The drawing under review shows one solid part. Ordinate dimensions are in mm from its lowest x, y, z. A direction names the side the tool comes from. Coordinates: 2 decimals unless noted, no trailing zeros. Order: outer loops, then holes, each group sorted by start corner. A loop starts at its lowest first (then second) coordinate and runs counter-clockwise, first axis right, second up. Notation, with made-up numbers: (14.25, 64) -> (47.25, 64) arc R32 ccw to (47.25, 96) -> close; hole circle Ø3 at (-0.75, 86.5). An arc over 180 degrees is marked (long way). Put each result on its own line as item: value.
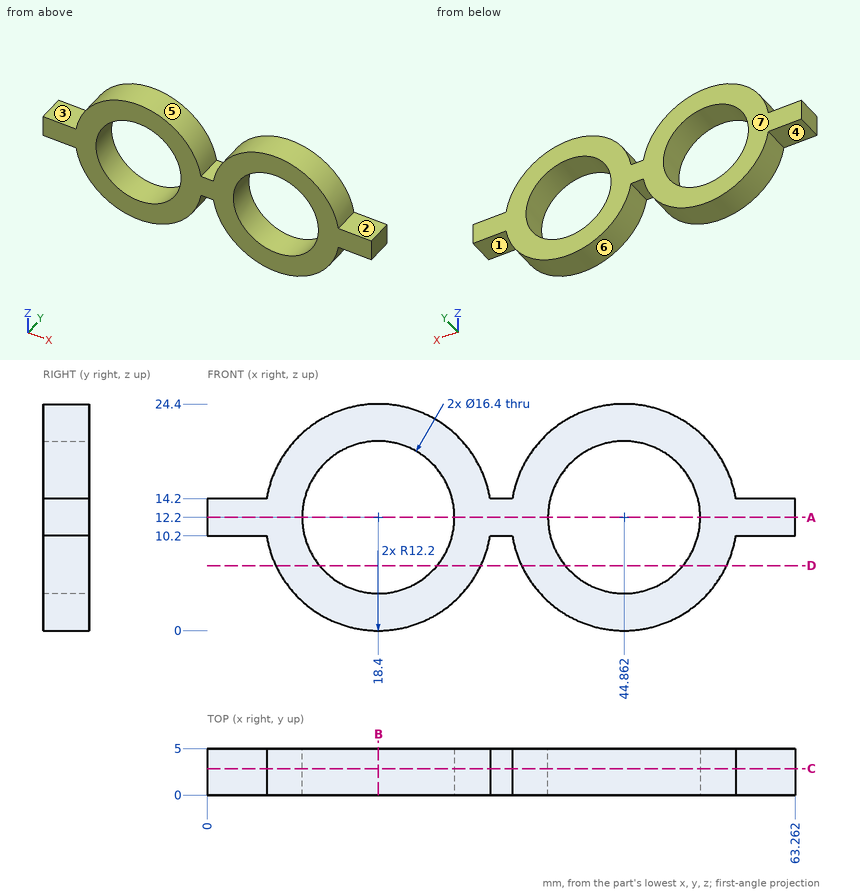
Item 1: For line 1 (X direction, y = 2.75, z = 6.5); line 2 (X direction, y = 0.2, z = 15.25); line 3 (X direction, y = 1.7, z = 13.5), list the stretches that pass through material, from the lowest coordinate up. Write a range as from..to.
Answers below:
line 1: 7.61..12.51, 24.29..29.19, 34.08..38.97, 50.76..55.65
line 2: 6.59..10.79, 26.01..30.21, 33.05..37.25, 52.47..56.67
line 3: 0..10.3, 26.5..36.77, 52.96..63.26
Item 2: Consider section A-A on z = 12.2. Write out the cut boundary in (x, y), and give its area (3 significant figures).
Answers below:
outline: (0, 0) -> (10.2, 0) -> (10.2, 5) -> (0, 5) -> close; (26.6, 0) -> (36.66, 0) -> (36.66, 5) -> (26.6, 5) -> close; (53.06, 0) -> (63.26, 0) -> (63.26, 5) -> (53.06, 5) -> close
area: 152 mm^2
Item 3: Consider section C-C on y = 2.85. Write out the cut boundary in (x, z).
Answers below:
outline: (0, 10.2) -> (6.37, 10.2) arc R12.2 ccw to (30.43, 10.2) -> (32.83, 10.2) arc R12.2 ccw to (56.9, 10.2) -> (63.26, 10.2) -> (63.26, 14.2) -> (56.9, 14.2) arc R12.2 ccw to (32.83, 14.2) -> (30.43, 14.2) arc R12.2 ccw to (6.37, 14.2) -> (0, 14.2) -> close; hole circle Ø16.4 at (18.4, 12.2); hole circle Ø16.4 at (44.86, 12.2)
Item 4: Consider section D-D on z = 7. Write out the cut boundary in (x, y), and give its area (3 significant figures).
Answers below:
outline: (7.36, 0) -> (12.06, 0) -> (12.06, 5) -> (7.36, 5) -> close; (24.74, 0) -> (29.44, 0) -> (29.44, 5) -> (24.74, 5) -> close; (33.83, 0) -> (38.52, 0) -> (38.52, 5) -> (33.83, 5) -> close; (51.2, 0) -> (55.9, 0) -> (55.9, 5) -> (51.2, 5) -> close
area: 93.9 mm^2
Item 5: Mouldability with a two-part tool opening along X and no side actions: class the marked faces 5, 6 and 7 as +X half, -X half, draft (parallel to the pull), parting line (faces both ways), or undercut.
Answers below:
face 5: undercut
face 6: undercut
face 7: draft
Item 6: For the marked faces 1, 2, 3 and 4, list the 3-axis set-ups (+Z, -Z, +X, -X, +Y, -Y) from which the entire face can be reached by the end or side of a thin tool; tool diameter is ignored.
Answers below:
face 1: -Z, +X, +Y, -Y
face 2: +Z, +X, +Y, -Y
face 3: +Z, -X, +Y, -Y
face 4: -Z, -X, +Y, -Y
Item 7: Consider section B-B on x = 18.4. Write out the cut boundary in (y, z), and give its area (3 significant figures).
Answers below:
outline: (0, 0) -> (5, 0) -> (5, 4) -> (0, 4) -> close; (0, 20.4) -> (5, 20.4) -> (5, 24.4) -> (0, 24.4) -> close
area: 40.0 mm^2
Item 8: For pin 1 Ø2 at (x, y) = (52.5, 1) entering from +Z; pin 2 Ø1.5 at (y, z) = (2.5, 5.5) entering from -X; pin 3 Ø1.9 at (x, y) = (31.5, 1.5) entering from +Z, all flat-tipped, find the tip position at first contact; note any pin that passes through.
Answers below:
pin 1: z = 22.44
pin 2: x = 7.75
pin 3: z = 14.2
